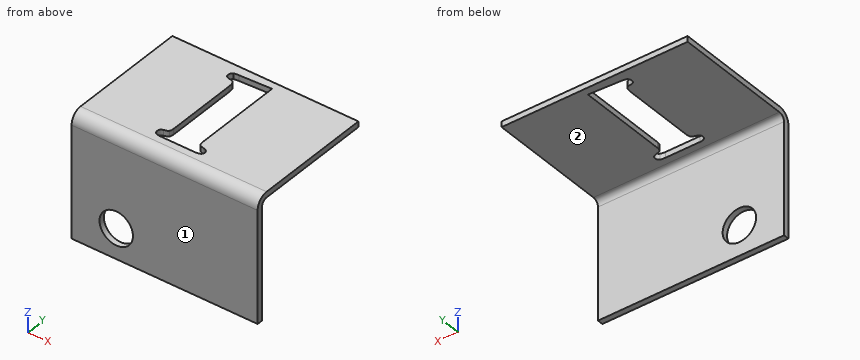
```python
from build123d import *

# Parameters (mm, degrees)
SKETCH1_W            = 50
SKETCH1_H            = 30
BASE_FLANGE1_DEPTH   = 1.51892
EDGE_FLANGE1_DEPTH   = 50
M8_CLEARANCE_HOLE1_D = 9
CUT_EXTRUDE1_DEPTH   = 55.277389816


# Sheet-metal steps are written as plain solids
with BuildPart() as part:
    # Sketch1 → Base-Flange1 (new body)
    with BuildSketch(Plane(origin=(0, 0, 0), x_dir=(1, 0, 0), z_dir=(0, 1, 0))):
        with Locations((0, 15)):
            Rectangle(SKETCH1_W, SKETCH1_H)
    extrude(amount=BASE_FLANGE1_DEPTH)

    # Edge-Flange1 section (across the edge) → Edge-Flange1 (add)
    with BuildSketch(Plane(origin=(-25, 1.51892, 1.5875), x_dir=(0, 0, -1), z_dir=(1, 0, 0))):
        with BuildLine():
            Line((-1.51892, 1.5875), (-1.51892, 33.48108))
            Line((-1.51892, 33.48108), (0, 33.48108))
            Line((0, 33.48108), (0, 1.5875))
            ThreePointArc((0, 1.5875), (0.464967985, 0.464967985), (1.5875, 0))
            Line((1.5875, 0), (1.5875, -1.51892))
            ThreePointArc((1.5875, -1.51892), (-0.609070647, -0.609070647), (-1.51892, 1.5875))
        make_face()
    extrude(amount=EDGE_FLANGE1_DEPTH)

    # M8 Clearance Hole1 (through all)
    with Locations(Plane(origin=(0, 1.51892, 0), x_dir=(1, 0, 0), z_dir=(0, 1, 0))):
        with Locations((-13, 21.89358)):
            Hole(M8_CLEARANCE_HOLE1_D / 2)

    # Sketch11 → Cut-Extrude1 (cut, through all)
    with BuildSketch(Plane.XY.offset(3.10642)):
        with BuildLine():
            Line((3.352683653, 33), (3.352683653, 8.876736111))
            add(Edge.make_bspline(
                [(3.352683653, 8.876736111), (3.353743072, 8.75248746), (3.355707508, 8.522098259), (3.431182496, 8.208449128), (3.514980812, 7.935424237), (3.62773347, 7.798723212), (3.680808653, 7.734375)],
                knots=[0, 0, 0, 0, 1.221894812, 2.265709648, 3.183630964, 4, 4, 4, 4], degree=3))
            add(Edge.make_bspline(
                [(3.680808653, 7.734375), (3.734677776, 7.676504164), (3.830117167, 7.573974975), (3.989367782, 7.479439012), (4.159797664, 7.433882679), (4.373058128, 7.390651398), (4.667575389, 7.304305676), (4.895720619, 7.252831146), (5.023690598, 7.223958333)],
                knots=[0, 0, 0, 0, 0.967781164, 1.714608312, 2.234126727, 3.127399629, 4.388716669, 6, 6, 6, 6], degree=3))
            add(Edge.make_bspline(
                [(5.023690598, 7.223958333), (5.181883466, 7.183631094), (5.472950316, 7.109431018), (5.825003123, 6.855284919), (6.042399674, 6.503977916), (6.06374242, 6.238622284), (6.074905875, 6.099826389)],
                knots=[0, 0, 0, 0, 1.155259645, 2.125619132, 3.019593567, 4, 4, 4, 4], degree=3))
            add(Edge.make_bspline(
                [(6.074905875, 6.099826389), (6.06732471, 6.015842007), (6.052127137, 5.847482842), (5.944064224, 5.60615586), (5.75097894, 5.402699673), (5.589337522, 5.298332742), (5.50372532, 5.243055556)],
                knots=[0, 0, 0, 0, 0.931770353, 1.867872026, 2.870733925, 4, 4, 4, 4], degree=3))
            add(Edge.make_bspline(
                [(5.50372532, 5.243055556), (5.423622762, 5.206171118), (5.246520526, 5.124621709), (4.930300382, 5.048945746), (4.546600649, 5.012201245), (4.268276747, 5.004272313), (4.118308653, 5)],
                knots=[0, 0, 0, 0, 0.744408225, 1.645844579, 2.731520362, 4, 4, 4, 4], degree=3))
            Line((4.118308653, 5), (3.37091282, 5))
            Line((3.37091282, 5), (-4.443323291, 5))
            Line((-4.443323291, 5), (-5.069191347, 5))
            add(Edge.make_bspline(
                [(-5.069191347, 5), (-5.200959456, 5.004230902), (-5.445003537, 5.012066838), (-5.780351524, 5.049107042), (-6.053589539, 5.123405658), (-6.200525, 5.206080373), (-6.266239958, 5.243055556)],
                knots=[0, 0, 0, 0, 1.278909849, 2.36863365, 3.270392795, 4, 4, 4, 4], degree=3))
            add(Edge.make_bspline(
                [(-6.266239958, 5.243055556), (-6.339681587, 5.298913512), (-6.481004414, 5.406400292), (-6.646771526, 5.611036077), (-6.740904198, 5.849325914), (-6.752565064, 6.016021642), (-6.758427458, 6.099826389)],
                knots=[0, 0, 0, 0, 1.071870055, 2.062586414, 3.025983099, 4, 4, 4, 4], degree=3))
            add(Edge.make_bspline(
                [(-6.758427458, 6.099826389), (-6.751201394, 6.238381888), (-6.737517447, 6.500763459), (-6.542576602, 6.842832855), (-6.244911058, 7.108230032), (-5.985928279, 7.183546642), (-5.846969125, 7.223958333)],
                knots=[0, 0, 0, 0, 1.041821617, 1.972890251, 2.912339053, 4, 4, 4, 4], degree=3))
            add(Edge.make_bspline(
                [(-5.846969125, 7.223958333), (-5.735122036, 7.252770415), (-5.537017037, 7.303802744), (-5.285346725, 7.389215809), (-5.104551332, 7.434528827), (-4.959644822, 7.480235759), (-4.824408418, 7.574602156), (-4.751821285, 7.676581079), (-4.710684402, 7.734375)],
                knots=[0, 0, 0, 0, 1.624637859, 2.877579422, 3.734891967, 4.248647568, 5.007466236, 6, 6, 6, 6], degree=3))
            add(Edge.make_bspline(
                [(-4.710684402, 7.734375), (-4.664199883, 7.799255117), (-4.563973926, 7.939144093), (-4.49111496, 8.20905769), (-4.431859524, 8.523582896), (-4.42746965, 8.752733909), (-4.425094125, 8.876736111)],
                knots=[0, 0, 0, 0, 0.793417505, 1.710699182, 2.761173524, 4, 4, 4, 4], degree=3))
            Line((-4.425094125, 8.876736111), (-4.425094125, 28.0234375))
            add(Edge.make_bspline(
                [(-4.425094125, 28.0234375), (-4.426531902, 28.191669086), (-4.429205189, 28.504465382), (-4.470592994, 28.937557572), (-4.538640115, 29.30004587), (-4.643358024, 29.592207067), (-4.770170391, 29.828354389), (-4.936878879, 30.004608948), (-5.143251784, 30.120886097), (-5.294711667, 30.152209661), (-5.373010791, 30.168402778)],
                knots=[0, 0, 0, 0, 1.573891919, 2.926368201, 4.067733782, 5.015207088, 5.82171764, 6.559095732, 7.255106106, 8, 8, 8, 8], degree=3))
            Line((-5.373010791, 30.168402778), (-6.132559402, 30.271701389))
            add(Edge.make_bspline(
                [(-6.132559402, 30.271701389), (-6.283854904, 30.300098434), (-6.559763459, 30.351884427), (-6.904178309, 30.569151507), (-7.122046768, 30.892299153), (-7.138654843, 31.143367481), (-7.147316347, 31.274305556)],
                knots=[0, 0, 0, 0, 1.161059911, 2.117355492, 3.018156337, 4, 4, 4, 4], degree=3))
            add(Edge.make_bspline(
                [(-7.147316347, 31.274305556), (-7.142422565, 31.381346659), (-7.132924891, 31.589088155), (-6.995811409, 31.871248407), (-6.805451884, 32.128706889), (-6.623451964, 32.249631783), (-6.52752468, 32.313368056)],
                knots=[0, 0, 0, 0, 1.003758752, 1.948058634, 2.918476655, 4, 4, 4, 4], degree=3))
            add(Edge.make_bspline(
                [(-6.52752468, 32.313368056), (-6.463477626, 32.342119574), (-6.312140707, 32.410056597), (-6.025881505, 32.457814765), (-5.664653043, 32.51745606), (-5.393638242, 32.534790019), (-5.245406625, 32.544270833)],
                knots=[0, 0, 0, 0, 0.641016437, 1.514659076, 2.640642126, 4, 4, 4, 4], degree=3))
            Line((-5.245406625, 32.544270833), (3.352683653, 33))
        make_face()
    extrude(amount=-CUT_EXTRUDE1_DEPTH, mode=Mode.SUBTRACT)


solid = part.part
```
The listing builds one solid part. Answer for the finished solid, in the listing's coordinates (mm). Face numbers are marked on the shaded views. A direction names the side the tool comes from. Round coordinates to 2 decimals unless told otherwise and drop trailing zeros. Loops run counter-clockwise (first coordinate to the right, second up) from the corner with the lowest first, then second, coordinate; pieces in that order, holes last.
Q1. Section D-D, the plane z = -5 is taken. Determine the outline of the cut face in (x, y).
Q2. Given pin 1 Ø5 at (x, y) = (14, 23) entering from -Z; pin 2 Ø1.5 at (x, z) = (-1, -17.5) entering from +Y, each flat-ended and moving along its own axis, determine where each tip first touches the part or whether it passes through.
Q3. Find the intervals of material crossed by line 1 (Y direction, x = -3, z = -22.5); line 2 (Z direction, x = 8, y = 18.5); line 3 (Z direction, x = -13, y = 0.3), in increasing order.
Q4. Section A-A, the plane y = 17.5 is taken. Determine the outline of the cut face in (x, z).
Q5. Section C-C, the plane x = 21.5 is taken. Determine the outline of the cut face in (y, z) (1 decimal).
Q6. Which of the six approach directions +Z, -Z, +X, -X, +Y, -Y give full straight-line access (tool end or side, diameter ignored) to the marked faces 1 and 2?
Q7. Section B-B, the plane x = -13 is taken. Determine the outline of the cut face in (y, z) (1 decimal), then the cut area to 3 significant figures.
Completed:
1. outline: (-25, 0) - (25, 0) - (25, 1.52) - (-25, 1.52) - close
2. pin 1: stops at z = 1.59
2. pin 2: stops at y = 1.52
3. line 1: y = 0 to 1.52
3. line 2: z = 1.59 to 3.11
3. line 3: z = -30 to -26.39, -17.39 to 1.33
4. outline: (-25, 1.59) - (-4.43, 1.59) - (-4.43, 3.11) - (-25, 3.11) - close; (3.35, 1.59) - (25, 1.59) - (25, 3.11) - (3.35, 3.11) - close
5. outline: (0, -30) - (1.5, -30) - (1.5, 0) arc R1.6 cw to (3.1, 1.6) - (35, 1.6) - (35, 3.1) - (3.1, 3.1) arc R3.1 ccw to (0, 0) - close
6. face 1: +Z, -Z, +X, -X, -Y
6. face 2: -Z, +X, -X, +Y
7. outline: (0, -30) - (1.5, -30) - (1.5, -26.4) - (0, -26.4) - close; (0, -17.4) - (1.5, -17.4) - (1.5, 0) arc R1.6 cw to (3.1, 1.6) - (35, 1.6) - (35, 3.1) - (3.1, 3.1) arc R3.1 ccw to (0, 0) - close
7. area: 85.9 mm2
